Geometry: final body of the model. Coordinates: model frame, mm. Give positions to 0.01 mm unless a question says otherwise; leave off trailing zeros. Order: outer loops, then holes, each group sorted by start corner. A loop starts at its lowest first (then second) coordinate and runs counter-clockwise, first axis right, second up. Notation, with made-up numbers: (35, 72) -> (73, 72) arc R22 ccw to (73, 104) -> close; hole circle Ø4 at (-38, 9.5). An arc over 180 degrees is marked (long way). One line per question, with ' | ' between items. Start each with the question number.
(1) Mould query, pull axis X, two halves, no side actions, for faces 1 (the face through (0, 2, 3.45)), 2 (the face through (3, 1.5, 1.7)), 3 (the face through (0, 2, 2)). Classes: +X half, -X half, draft (parallel to the pull), parting line (faces both ways), or undercut.
(2) Section C-C (y = 1.3). Return loops of the section in (x, z), then the cut area to 3 significant figures.
(3) First-contact query: pin 1 Ø3.5 at (x, z) = (0, 0) entering from -Y; pin 2 Ø1.5 at (y, z) = (1.5, 1) entering from -X. Flat tips, straight axial feed; report the tip coordinate or a pass-through.
(4) Section A-A (x = 0). Return loops of the section in (y, z), then the cut area to 3 significant figures.
(5) Section B-B (z = -0.25). Return loops of the section in (x, y).
(6) Section D-D (z = 2.25). Return loops of the section in (x, y).
(7) Ray query, L1, parallel to Z at x = 0, y = 1.35; L2, parallel to Z at x = -1.75, y = 2.7; L3, parallel to X at y = 0.45, z = -1. Return the intervals inside material, ascending.
Autodesk Inventor part; units mm, degrees
ref_plane "YZ Plane" through (0, 0, 0) normal (1, 0, 0) x (0, 1, 0)
ref_plane "XZ Plane" through (0, 0, 0) normal (0, 1, 0) x (-1, 0, 0)
ref_plane "XY Plane" through (0, 0, 0) normal (0, 0, 1) x (1, 0, 0)
sketch "Sketch1" plane through (0, 0, 0) normal (0, 1, 0) x (-1, 0, 0)
  circle A0 centre (0, 0) radius 2
  line L0 (-1.9919, -3.45) -> (-3.9837, 0)
  line L1 (-3.9837, 0) -> (-1.9919, 3.45)
  line L2 (-1.9919, 3.45) -> (1.9919, 3.45)
  line L3 (1.9919, 3.45) -> (3.9837, 0)
  line L4 (3.9837, 0) -> (1.9919, -3.45)
  line L5 (1.9919, -3.45) -> (-1.9919, -3.45)
  line L6 (0, 0) -> (9.6963, 0) construction
  dimension "d0" = 6.9
  dimension "d1" = 4
extrude "Extrusion1" add sketch "Sketch1" along normal blind 3.06
thread "Thread1"
properties part number "M4 nut"
Response:
1) face 1: draft | face 2: +X half | face 3: undercut
2) outline: (-3.98, 0) -> (-1.99, -3.45) -> (1.99, -3.45) -> (3.98, 0) -> (1.99, 3.45) -> (-1.99, 3.45) -> close; hole circle Ø4 at (0, 0) | area: 28.7 mm^2
3) pin 1: passes through | pin 2: stops at x = -3.84
4) outline: (0, -3.45) -> (3.06, -3.45) -> (3.06, -2) -> (0, -2) -> close; (0, 2) -> (3.06, 2) -> (3.06, 3.45) -> (0, 3.45) -> close | area: 8.87 mm^2
5) outline: (-3.84, 0) -> (-1.98, 0) -> (-1.98, 3.06) -> (-3.84, 3.06) -> close; (1.98, 0) -> (3.84, 0) -> (3.84, 3.06) -> (1.98, 3.06) -> close
6) outline: (-2.68, 0) -> (2.68, 0) -> (2.68, 3.06) -> (-2.68, 3.06) -> close
7) L1: z = -3.45 to -2, 2 to 3.45 | L2: z = -3.45 to -0.97, 0.97 to 3.45 | L3: x = -3.41 to -1.73, 1.73 to 3.41
